The listing builds one solid part. Answer for the finished solid, in the listing's coordinates (mm). Face numbers are marked on the shaded views. A direction names the side the tool comes from. Round coordinates to 2 decimals unless told otherwise and drop trailing zeros. Loops run counter-clockwise (first coordinate to the right, second up) from the corner with the lowest first, then second, coordinate; pieces in that order, holes last. Notation, with made-up numbers: M 74.5,9 L 101.5,9 A23 cw 101.5,40 Z; hole C 11,89 d5. An arc over 180 degrees is marked long. Put each result on its own line as item: value. Start each with the question number.
(1) Section B-B, the plane x = 0 is taken. Count the separate pieces of the cut face and the enclosed holes in it, then the cut area to 3 significant figures.
(2) Section C-C, the plane y = 0 is taken. Determine the outline of the cut face in (x, z), then the cut area to 4 significant figures.
(3) Section D-D, the plane x = -21 is taken. Determine the outline of the cut face in (y, z).
(4) Which of the six approach directions +Z, -Z, +X, -X, +Y, -Y give full straight-line access (tool end or side, diameter ignored) to the marked faces 1, 2, 3, 4 and 5?
(5) Straight lines are drawn through the part: line 1 (Y direction, x = 0, z = 0.4); line 2 (X direction, y = 0, z = 2.25); line 3 (Y direction, x = 0, z = 1.8). For each, find the intervals that lie inside material, in ascending order.
(6) Section A-A, the plane y = 42.75 is taken. Determine the outline of the cut face in (x, z), then the cut area to 3 significant figures.
(7) Determine the mould class of the marked faces 6, 7 and 8 for opening direction Y: released by +Y, released by -Y, zero draft, split by the parting line, or undercut.
(8) Flat-ended cylindrical pins translate along their axes: P1, Ø10, axis at x = -1.5, y = 44.5, coming from the +Z side; P2, Ø1.6, axis at x = 17.54, y = 10.12, coming from the +Z side; P3, Ø3, axis at x = -1, y = -24.5, coming from the +Z side; P4, Ø23, axis at x = -8, y = -3.5, coming from the +Z side. Find the tip coordinate at first contact, or state that the pin passes through.
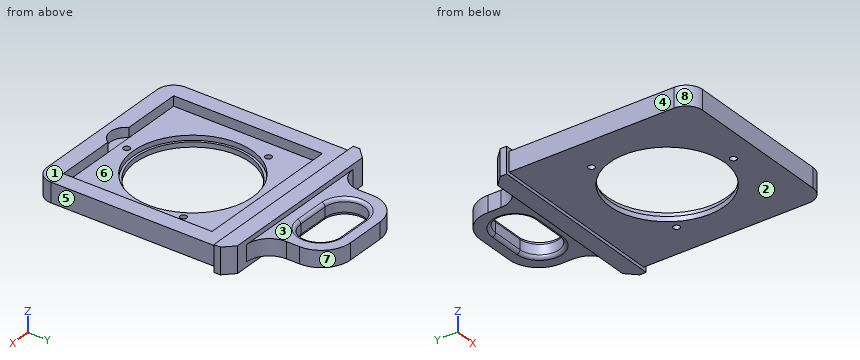
```python
from build123d import *

# Parameters (mm, degrees)
SKETCH_W        = 55.5
SKETCH_H        = 55.5
SKETCH_R        = 18.25
PAD_DEPTH       = 6
SKETCH001_W     = 57.5
SKETCH001_H     = 8
PAD001_DEPTH    = 5
SKETCH002_W     = 30
SKETCH002_H     = 5
PAD002_DEPTH    = 20
FILLET_R        = 5
POCKET_DEPTH    = 6
FILLET001_R     = 9
FILLET002_R     = 7
CHAMFER_SIZE    = 3
SKETCH004_R     = 18.25
SKETCH004_R_2   = 17.5
PAD003_DEPTH    = 1.5
SKETCH005_W     = 45.5
SKETCH005_H     = 45.5
POCKET001_DEPTH = 3
SKETCH006_R     = 1
POCKET002_DEPTH = 6
FILLET003_R     = 1
FILLET004_R     = 1
SKETCH007_R     = 5
POCKET003_DEPTH = 2.999


with BuildPart() as part:
    # Sketch → Pad (new body)
    with BuildSketch(Plane.XY):
        Rectangle(SKETCH_W, SKETCH_H)
        Circle(SKETCH_R, mode=Mode.SUBTRACT)
    extrude(amount=PAD_DEPTH)

    # Sketch001 → Pad001 (new body)
    with BuildSketch(Plane(origin=(0, 27.75, 0), x_dir=(-1, 0, 0), z_dir=(0, 1, 0))):
        with Locations((0, 3)):
            Rectangle(SKETCH001_W, SKETCH001_H)
    extrude(amount=PAD001_DEPTH)

    # Sketch002 → Pad002 (new body)
    with BuildSketch(Plane(origin=(0, 32.75, 0), x_dir=(-1, 0, 0), z_dir=(0, 1, 0))):
        with Locations((0, 3)):
            Rectangle(SKETCH002_W, SKETCH002_H)
    extrude(amount=PAD002_DEPTH)

    # Fillet
    fillet_edges = [part.edges().sort_by_distance(p)[0] for p in [
        (-27.75, -27.75, 3),
        (27.75, -27.75, 3),
    ]]
    fillet(fillet_edges, radius=FILLET_R)

    # Sketch003 → Pocket (cut)
    with BuildSketch(Plane(origin=(0, 0, 0.5), x_dir=(1, 0, 0), z_dir=(0, 0, -1))):
        with BuildLine():
            ThreePointArc((-5, -36.75), (-11, -42.75), (-5, -48.75))
            Line((-5, -48.75), (5, -48.75))
            ThreePointArc((5, -48.75), (11, -42.75), (5, -36.75))
            Line((-5, -36.75), (5, -36.75))
        make_face()
    extrude(amount=-POCKET_DEPTH, mode=Mode.SUBTRACT)

    # Fillet001
    fillet001_edges = [part.edges().sort_by_distance(p)[0] for p in [
        (15, 52.75, 3),
        (-15, 52.75, 3),
    ]]
    fillet(fillet001_edges, radius=FILLET001_R)

    # Fillet002
    fillet002_edges = [part.edges().sort_by_distance(p)[0] for p in [
        (15, 32.75, 3),
        (-15, 32.75, 3),
    ]]
    fillet(fillet002_edges, radius=FILLET002_R)

    # Chamfer
    chamfer_edges = [part.edges().sort_by_distance(p)[0] for p in [
        (-28.75, 32.75, 3),
        (28.75, 32.75, 3),
    ]]
    chamfer(chamfer_edges, length=CHAMFER_SIZE)

    # Sketch004 → Pad003 (new body)
    with BuildSketch(Plane(origin=(0, 0, 0), x_dir=(1, 0, 0), z_dir=(0, 0, -1))):
        Circle(SKETCH004_R)
        Circle(SKETCH004_R_2, mode=Mode.SUBTRACT)
    extrude(amount=-PAD003_DEPTH)

    # Sketch005 → Pocket001 (cut)
    with BuildSketch(Plane.XY.offset(6)):
        Rectangle(SKETCH005_W, SKETCH005_H)
    extrude(amount=-POCKET001_DEPTH, mode=Mode.SUBTRACT)

    # Sketch006 → Pocket002 (cut)
    with BuildSketch(Plane.XY.offset(3)):
        with Locations((-17.537014, 10.125)):
            Circle(SKETCH006_R)
        with Locations((17.537014, 10.125)):
            Circle(SKETCH006_R)
        with Locations((0, -20.25)):
            Circle(SKETCH006_R)
    extrude(amount=-POCKET002_DEPTH, mode=Mode.SUBTRACT)

    # Fillet003
    fillet003_edges = [part.edges().sort_by_distance(p)[0] for p in [
        (0, 48.75, 5.5),
    ]]
    fillet(fillet003_edges, radius=FILLET003_R)

    # Fillet004
    fillet004_edges = [part.edges().sort_by_distance(p)[0] for p in [
        (0, 36.75, 0.5),
    ]]
    fillet(fillet004_edges, radius=FILLET004_R)

    # Sketch007 → Pocket003 (cut)
    with BuildSketch(Plane.XY.offset(6)):
        with Locations((0, -20.25)):
            Circle(SKETCH007_R)
    extrude(amount=-POCKET003_DEPTH, mode=Mode.SUBTRACT)


solid = part.part
```
Recorded:
1. separate pieces: 4
1. enclosed holes: 0
1. area: 155 mm²
2. outline: M -27.75,0 L -17.5,0 L -17.5,1.5 L -18.25,1.5 L -18.25,3 L -22.75,3 L -22.75,6 L -27.75,6 Z; M 17.5,0 L 27.75,0 L 27.75,6 L 22.75,6 L 22.75,3 L 18.25,3 L 18.25,1.5 L 17.5,1.5 Z
2. area: 89.25 mm²
3. outline: M -27.75,0 L 27.75,0 L 27.75,-1 L 32.75,-1 L 32.75,0.5 L 32.82,0.5 L 32.82,5.5 L 32.75,5.5 L 32.75,7 L 27.75,7 L 27.75,6 L 22.75,6 L 22.75,3 L -22.75,3 L -22.75,6 L -27.75,6 Z
4. face 1: +Z, +X, -X, -Y
4. face 2: -Z, +X, -X, -Y
4. face 3: +Z, +X, -X, +Y
4. face 4: +Z, -Z, -X, -Y
4. face 5: +Z, -Z, +X, -Y
5. line 1: y = -27.75 to -21.25, -19.25 to -17.5, 17.5 to 32.75
5. line 2: x = -27.75 to -18.25, 18.25 to 27.75
5. line 3: y = -27.75 to -21.25, -19.25 to -18.25, 18.25 to 36.75, 48.75 to 52.75
6. outline: M -15,0.5 L -12,0.5 A1 ccw -11,1.5 L -11,4.5 A1 ccw -12,5.5 L -15,5.5 Z; M 11,1.5 A1 ccw 12,0.5 L 15,0.5 L 15,5.5 L 12,5.5 A1 ccw 11,4.5 Z
6. area: 39.1 mm²
7. face 6: undercut
7. face 7: released by +Y
7. face 8: released by -Y
8. P1: stops at z = 5.47
8. P2: passes through
8. P3: stops at z = 6
8. P4: stops at z = 3
